Autodesk Inventor part; units mm, degrees
ref_plane "YZ Plane" through (0, 0, 0) normal (1, 0, 0) x (0, 1, 0)
ref_plane "XZ Plane" through (0, 0, 0) normal (0, 1, 0) x (-1, 0, 0)
ref_plane "XY Plane" through (0, 0, 0) normal (0, 0, 1) x (1, 0, 0)
sketch "Esboço5" plane through (0, 0, 0) normal (0, 0, 1) x (1, 0, 0)
  line L0 (0, 50) -> (0, -50)
  line L1 (0, 0) -> (-3.5, 0)
  line L2 (-3.5, 0) -> (-3.5, 16)
  line L3 (-3.5, 16) -> (0, 16)
  line L4 (0, 16) -> (0, 0)
  line L5 (0, 16) -> (0, 21)
  line L6 (0, 21) -> (-0.4, 21)
  line L7 (-0.4, 21) -> (-0.4, 16)
  line L8 (-0.4, 16) -> (0, 16)
  line L9 (-2.7292, 0) -> (-2.7292, -5)
  line L10 (-0.7292, 0) -> (-0.7292, -5)
  line L11 (-0.7292, 0) -> (-0.7292, -5)
  line L12 (-0.7292, -5) -> (-1.0292, -5)
  line L13 (-1.0292, -5) -> (-1.0292, 0)
  line L14 (-1.0292, 0) -> (-0.7292, 0)
  line L15 (-2.7292, 0) -> (-2.7292, -5)
  line L16 (-2.7292, -5) -> (-2.4292, -5)
  line L17 (-2.4292, -5) -> (-2.4292, 0)
  line L18 (-2.4292, 0) -> (-2.7292, 0)
  point P0 (-1.0292, 0)
  dimension "d22" = 100
  dimension "d23" = 3.5
  dimension "d24" = 16
  dimension "d25" = 5
  dimension "d26" = 0.4
  dimension "d37" = 5
  dimension "d38" = 5
  dimension "d39" = 2
  dimension "d40" = 1.4584
  dimension "d41" = 0
  dimension "d42" = 21
  dimension "d43" = 0.8
  dimension "d44" = 5
  dimension "d45" = 5
  dimension "d46" = 0.3
  dimension "d47" = 5
  dimension "d48" = 0.3
revolve "Revolução6" add sketch "Esboço5" angle 360 mid plane about axis through (0, 50, 0) along (0, -1, 0) contours L0 L3 L7 L6 | L0 L1 L2 L3
revolve "Revolução7" add sketch "Esboço5" angle 360 mid plane about axis through (-0.7292, 0, 0) along (0, -1, 0) contours L10 L12 L13 L1
revolve "Revolução8" add sketch "Esboço5" angle 360 mid plane about axis through (-2.4292, -5, 0) along (0, 1, 0) contours L17 L16 L9 L1
fillet "Arredondamento4" radius 0.1 1 edges at (-0.4, 21, 0)
fillet "Arredondamento5" radius 0.3 2 edges at (-3.5, 16, 0) (-3.5, 0, 0)
properties part number "Motor"
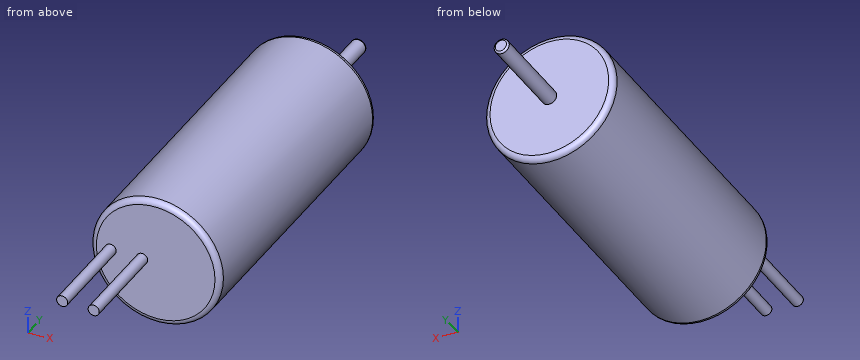
Read the model definition and answer for the solid it produces. Units are mm, in the model's axes. Round coordinates to 2 decimals unless told otherwise and drop trailing zeros. Loops run counter-clockwise (first coordinate to the right, second up) from the corner with the lowest first, then second, coordinate; pieces in that order, holes last. Notation, with made-up numbers: (54.25, 49.5) - (62.25, 49.5) arc R24 cw to (62.25, 88.5) - close; hole circle Ø11 at (82.5, -8.5). An arc over 180 degrees is marked (long way). One line per question, with ' | ' between items. Start each with the question number.
Q1. Section B-B on x = 0 is taken. Give the vertices of the cut face in (y, z), plus the area to 3 significant figures.
Q2. Section C-C on y = 14.5 is taken. Give the vertices of the cut face in (x, z), plus the area to 3 significant figures.
Q3. Find the intervals of material crossed by L1, parallel to Y at x = 0.25, z = -1.25; L2, parallel to X at y = -2.25, z = 0.25; L3, parallel to Z at x = 1, y = 12.75, in increasing order.
Q4. Section A-A on z = 0 is taken. Give the vertices of the cut face in (x, y).
Q5. Flat-ended cylindrical pins translate along their axes: pin 1 (3 mm diameter, centred on x = 1, z = 0, fed in from -Y); pin 2 (1 mm diameter, centred on x = -3, z = -1.5, fed in from +Y); pin 3 (1 mm diameter, centred on x = -1.5, z = -2.5, fed in from -Y). Find the tip coordinate at first contact, or state that the pin passes through.
Established:
1) outline: (0, -3.2) arc R0.3 ccw to (0.3, -3.5) - (15.7, -3.5) arc R0.3 ccw to (16, -3.2) - (16, -0.4) - (20.9, -0.4) arc R0.1 ccw to (21, -0.3) - (21, 0.3) arc R0.1 ccw to (20.9, 0.4) - (16, 0.4) - (16, 3.2) arc R0.3 ccw to (15.7, 3.5) - (0.3, 3.5) arc R0.3 ccw to (0, 3.2) - close | area: 116 mm²
2) outline: circle Ø7 at (0, 0) | area: 38.5 mm²
3) L1: 0 to 16 | L2: -2.6 to -2.26, -0.9 to -0.56 | L3: -3.35 to 3.35
4) outline: (-3.5, 0.3) arc R0.3 ccw to (-3.2, 0) - (-2.73, 0) - (-2.73, -5) - (-2.13, -5) - (-2.13, 0) - (-1.03, 0) - (-1.03, -5) - (-0.43, -5) - (-0.43, 0) - (3.2, 0) arc R0.3 ccw to (3.5, 0.3) - (3.5, 15.7) arc R0.3 ccw to (3.2, 16) - (0.4, 16) - (0.4, 20.9) arc R0.1 ccw to (0.3, 21) - (-0.3, 21) arc R0.1 ccw to (-0.4, 20.9) - (-0.4, 16) - (-3.2, 16) arc R0.3 ccw to (-3.5, 15.7) - close
5) pin 1: y = -5 | pin 2: y = 16 | pin 3: y = 0
